from build123d import *
from build123d.topology import SkipClean

# Parameters (mm, degrees)
SKETCH1_R           = 4.7625
SKETCH1_R_2         = 11.1125
BOSS_EXTRUDE3_DEPTH = 76.2


with BuildPart() as part:
    # Sketch1 → Boss-Extrude3 (new body)
    with BuildSketch(Plane.YZ):
        with BuildLine():
            Line((0, -14.2875), (0, 0))
            Line((0, 0), (-25.4, 0))
            Line((-25.4, 0), (-88.9, 76.2))
            Line((-88.9, 76.2), (-101.6, 76.2))
            Line((-101.6, 76.2), (-101.6, 0))
            Line((-101.6, 0), (-72.270606325, -50.8))
            Line((-72.270606325, -50.8), (0, -50.8))
            Line((0, -50.8), (0, -42.8625))
            ThreePointArc((0, -42.8625), (-14.2875, -28.575), (0, -14.2875))
        make_face()
        with Locations(Location((-63.5, -25.4, 0), (0, 0, 90))):
            Circle(SKETCH1_R, mode=Mode.SUBTRACT)
        with Locations(Location((-63.5, 0, 0), (0, 0, 90))):
            Circle(SKETCH1_R, mode=Mode.SUBTRACT)
        with Locations(Location((-76.2, 25.4, 0), (0, 0, 90))):
            Circle(SKETCH1_R_2, mode=Mode.SUBTRACT)
    extrude(amount=BOSS_EXTRUDE3_DEPTH)

    # Mirror1: part across plane


with BuildPart() as part_1:
    with SkipClean():  # the faces are left unmerged after this step: merging them gives an invalid solid
        add(part.part)
        add(part.part.mirror(Plane(origin=(76.2, 0, 0), x_dir=(0, 0, 1), z_dir=(0, -1, 0))))


solid = part_1.part
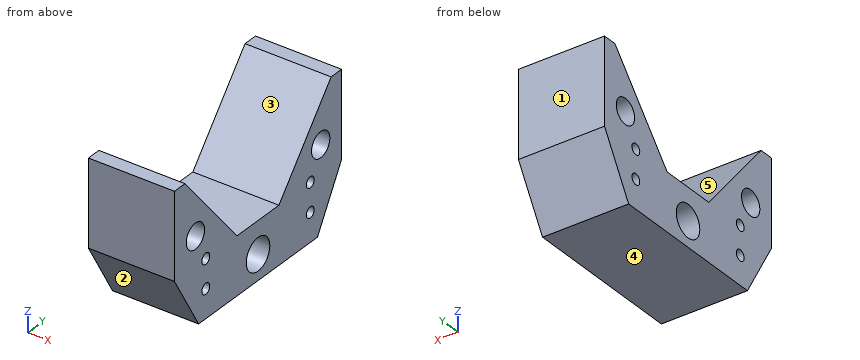
The model under review builds one solid part; all positions refer to its coordinate system, in mm. Face numbers are marked on the shaded views. A direction names the side the tool comes from. Coordinates: 2 decimals unless noted, no trailing zeros. Write each loop counter-clockwise with the first axis right and the second up, starting at its lowest first coordinate (ties: lowest second). Pieces come first, ordered by that corner, then holes. Notation, with made-up numbers: (35, 52.5) - (86, 52.5) arc R19 cw to (86, 70.5) - close; hole circle Ø11 at (61, 25). An arc over 180 degrees is marked (long way). Answer as a JSON object with one key per item and string values. Group by question number.
1. Mouldability with a two-part tool opening along Y and no side actions: class the marked faces 1, 2 and 3 as pulls with the +Y half, pulls with the -Y half, needs draft (parallel to the pull), parting line crosses it, or undercut.
2. To check wall thickness, follow probe 1 along Z at (x, y) = (57, 63); probe 2 along Y at (x, z) = (46, -25); probe 3 along Y at (x, z) = (48, 25). State the ranges of each line that lie inside material, in increasing order.
3. Add section D-D (y = -42.5). Give the boundary of the cut face in (x, z).
4. Add section B-B (z = -25.4). Give the boundary of the cut face in (x, y).
5. Add section C-C (x = 7). Give the boundary of the cut face in (y, z) (1 decimal), plus the area to 3 significant figures.
6. Add section A-A (y = 0). Give the boundary of the cut face in (x, z), plus the area to 3 significant figures.
7. Clearance check with flat-ended pins moving along their axes: pin 1 Ø12 at (x, y) = (9.5, -3) entering from +Z; pin 2 Ø2 at (x, z) = (36, -4.5) entering from -Y; pin 3 Ø1.5 at (x, y) = (27, -72.5) entering from +Z. State where each tip first meets the part, or that it passes through.
8. Machinability: for the marked faces 4 and 5, which of the approach directions +Z, -Z, +X, -X, +Y, -Y give a long, thin tool a straight path to every point of the face, cutting with its end or side? Answer none if there is none.
Findings:
{
 "1": {"face 1": "pulls with the +Y half", "face 2": "pulls with the -Y half", "face 3": "undercut"},
 "2": {"probe 1": "-50.8 to -30.14, -20.66 to -4.74, 4.74 to 45.12", "probe 2": "-87.17 to -68.25, -58.75 to -13.83, 13.83 to 58.75, 68.25 to 87.17", "probe 3": "-101.6 to -87.31, -65.09 to -46.23, 46.23 to 65.09, 87.31 to 101.6"},
 "3": {"outline": "(0, -50.8) - (76.2, -50.8) - (76.2, 20.52) - (0, 20.52) - close"},
 "4": {"outline": "(0, -86.94) - (76.2, -86.94) - (76.2, -68.26) - (0, -68.26) - close; (0, -58.74) - (76.2, -58.74) - (76.2, -13.93) - (0, -13.93) - close; (0, 13.93) - (76.2, 13.93) - (76.2, 58.74) - (0, 58.74) - close; (0, 68.26) - (76.2, 68.26) - (76.2, 86.94) - (0, 86.94) - close"},
 "5": {"outline": "(-101.6, 0) - (-72.3, -50.8) - (72.3, -50.8) - (101.6, 0) - (101.6, 76.2) - (88.9, 76.2) - (25.4, 0) - (-25.4, 0) - (-88.9, 76.2) - (-101.6, 76.2) - close; hole circle Ø22.2 at (-76.2, 25.4); hole circle Ø9.5 at (-63.5, -25.4); hole circle Ø9.5 at (-63.5, 0); hole circle Ø28.6 at (0, -28.6); hole circle Ø9.5 at (63.5, -25.4); hole circle Ø9.5 at (63.5, 0); hole circle Ø22.2 at (76.2, 25.4)", "area": "13,900 mm²"},
 "6": {"outline": "(0, -50.8) - (76.2, -50.8) - (76.2, -42.86) - (0, -42.86) - close; (0, -14.29) - (76.2, -14.29) - (76.2, 0) - (0, 0) - close", "area": "1,690 mm²"},
 "7": {"pin 1": "z = 0", "pin 2": "y = -99.58", "pin 3": "z = 57.42"},
 "8": {"face 4": "-Z, +X, -X, +Y, -Y", "face 5": "+Z, +X, -X"}
}
